```python
from build123d import *

# Parameters (mm, degrees)
F0_R        = 12.7
F1_DEPTH    = 6.35
F2_R        = 12.7
F3_DEPTH    = 63.5
F3_FACE_R   = 19.05
F3_FACE_R_2 = 12.7
F4_R        = 19.05
F4_R_2      = 4.7625
F5_DEPTH    = 25.4


with BuildPart() as f1:
    # F0 (on Top) → F1 (new body)
    with BuildSketch(Plane.XY):
        with BuildLine():
            Line((0, 9.398), (0, 0))
            Line((0, 0), (101.6, 0))
            Line((101.6, 0), (101.6, 9.4413837329))
            Line((101.6, 9.4413837329), (85.851973152, 9.4413837329))
            ThreePointArc((85.851973152, 9.4413837329), (76.199973152, 19.0933837329), (85.851973152, 28.7453837329))
            Line((85.851973152, 28.7453837329), (101.6, 28.7453837329))
            Line((101.6, 28.7453837329), (101.6, 38.1))
            Line((101.6, 38.1), (50.7999907375, 38.1))
            Line((50.7999907375, 38.1), (-1.85251e-05, 38.1))
            Line((-1.85251e-05, 38.1), (-1.85251e-05, 28.702))
            Line((-1.85251e-05, 28.702), (15.748, 28.702))
            ThreePointArc((15.748, 28.702), (25.4, 19.05), (15.748, 9.398))
            Line((15.748, 9.398), (0, 9.398))
        make_face()
        with Locations((50.8, 19.05)):
            Circle(F0_R, mode=Mode.SUBTRACT)
    extrude(amount=F1_DEPTH)

    # F2 (on face) → F3 (join)
    with BuildSketch(Plane(origin=(0, 0, 0), x_dir=(1, 0, 0), z_dir=(0, 0, -1))):
        with BuildLine():
            ThreePointArc((50.8, -38.1), (64.2703841816, -32.5203841816), (69.85, -19.05))
            ThreePointArc((69.85, -19.05), (64.2703841816, -5.5796158184), (50.8, 0))
            ThreePointArc((50.8, 0), (31.75, -19.05), (50.8, -38.1))
        make_face()
        with Locations((50.8, -19.05)):
            Circle(F2_R, mode=Mode.SUBTRACT)
    extrude(amount=F3_DEPTH)

    # F3_face (on face) + F4 (on Top) → F5 (join)
    with BuildSketch(Plane(origin=(50.8, 19.05, -63.5), x_dir=(1, 0, 0), z_dir=(0, 0, -1))):
        Circle(F3_FACE_R)
        Circle(F3_FACE_R_2, mode=Mode.SUBTRACT)
    with BuildSketch(Plane.XY):
        with Locations((50.8, 19.05)):
            Circle(F4_R)
        with Locations((50.8, 19.05)):
            Circle(F4_R_2, mode=Mode.SUBTRACT)
    extrude(amount=F5_DEPTH, dir=(0, 0, -1))


solid = f1.part
```
CAD build for the part. Positions are in the model's coordinates, mm. A direction names the side the tool comes from. Give positions to 0.01 mm unless a question says otherwise; leave off trailing zeros. Order: outer loops, then holes, each group sorted by start corner. A loop starts at its lowest first (then second) coordinate and runs counter-clockwise, first axis right, second up.
(1) Flat gauge pins, fed straight in: pin 1 (11 mm diameter, centred on x = 50.8, y = 19.05, fed in from -Z); pin 2 (4 mm diameter, centred on x = 36.5, z = -15.5, fed in from +Y); pin 3 (3 mm diameter, centred on x = 56.5, z = -13.5, fed in from -Y). Where does each tip first touch, or does it go through?
(2) Saw through at A-A, the plane x = 8. Give the cut face in (y, z), then the cut area to 3 significant figures.
(3) Mould opens along Y. For faces 5 (the flat face through (52, 38.1, 3)), 6 (the cylindrical face through (31.77, 18.21, -43.83)), 7 (the flat face through (101.6, 33, 3)), 8 (the cylindrical face through (47.29, 22.27, -12.52)) say: released by +Y, released by -Y, zero draft, split by the parting line, or undercut.
(4) Saw through at D-D, the plane y = 33. Give the cut face in (x, z).
(5) Saw through at B-B, the plane y = 19.05. Give the cut face in (x, z), then the cut area to 3 significant figures.
(6) Drill centre lines: L1, parallel to Y at x = 50, z = -46; L2, parallel to X at y = 19, z = 2; L3, parallel to Z at x = 83.5, y = 6. Where is each one in solid material? Low to high.
(7) Tool access for faces 1 (the flat face through (94, 28.745, 3)), 2 (the cylindrical face through (41.44, 10.467, 3.219)), 3 (the flat face through (8, 9.398, 3)), 4 (the flat face through (56, 19, -25.4)): list every direction of +Z, -Z, +X, -X, +Y, -Y with a clear straight run to the whole face (end or side of a thin tool).
(8) Saw through at C-C, the plane z = -35. Give the cut face in (x, y).
Results found:
1. pin 1: stops at z = -25.4
1. pin 2: stops at y = 33.6
1. pin 3: stops at y = 0.47
2. outline: (0, 0) - (9.4, 0) - (9.4, 6.35) - (0, 6.35) - close; (28.7, 0) - (38.1, 0) - (38.1, 6.35) - (28.7, 6.35) - close
2. area: 119 mm2
3. face 5: released by +Y
3. face 6: split by the parting line
3. face 7: zero draft
3. face 8: undercut
4. outline: (0, 0) - (37.83, 0) - (37.83, -88.9) - (63.77, -88.9) - (63.77, 0) - (101.6, 0) - (101.6, 6.35) - (0, 6.35) - close
5. outline: (25.4, 0) - (31.75, 0) - (31.75, -88.9) - (38.1, -88.9) - (38.1, -25.4) - (46.04, -25.4) - (46.04, 0) - (38.1, 0) - (38.1, 6.35) - (25.4, 6.35) - close; (55.56, -25.4) - (63.5, -25.4) - (63.5, -88.9) - (69.85, -88.9) - (69.85, 0) - (76.2, 0) - (76.2, 6.35) - (63.5, 6.35) - (63.5, 0) - (55.56, 0) - close
5. area: 1,690 mm2
6. L1: y = 0.02 to 6.38, 31.72 to 38.08
6. L2: x = 25.4 to 38.1, 63.5 to 76.2
6. L3: z = 0 to 6.35
7. face 1: +Z, -Z, +X
7. face 2: +Z
7. face 3: +Z, -Z, -X
7. face 4: -Z
8. outline: circle Ø38.1 at (50.8, 19.05); hole circle Ø25.4 at (50.8, 19.05)
